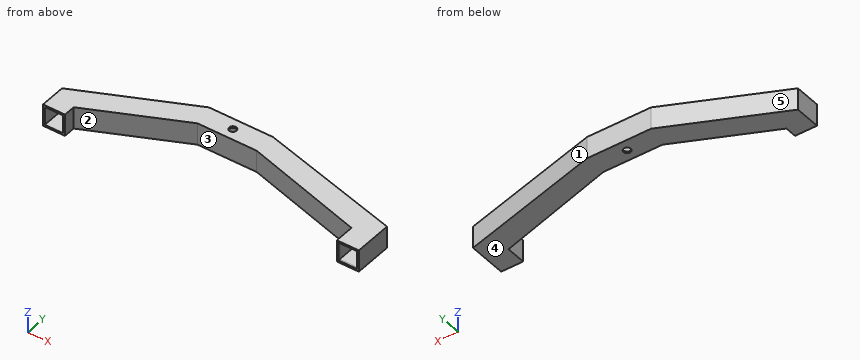
from build123d import *

# Parameters (mm, degrees)
BOSS_EXTRUDE1_DEPTH = 12
SHELL1_T            = -1
SKETCH2_W           = 10
SKETCH2_H           = 10
CUT_EXTRUDE1_DEPTH  = 12
SKETCH3_R           = 2
CUT_EXTRUDE2_DEPTH  = 12
CUT_EXTRUDE3_REACH  = 43.63
SKETCH5_W           = 0.21800788
SKETCH5_H           = 12


with BuildPart() as part:
    # Sketch1 → Boss-Extrude1 (new body)
    with BuildSketch(Plane.XY):
        Polygon((82.939086493, -35.63), (82.939086493, -24.776717085), (17.5, -6), (-14.870410096, -6), (-65.342905627, -29.23610302), (-65.342905627, -35.63), (-77.342905627, -35.63), (-77.342905627, -21.549973615), (-17.5, 6), (17.5, 6), (95.157094373, -14.812940234), (95.157094373, -35.63), align=None)
    extrude(amount=BOSS_EXTRUDE1_DEPTH)

    # Shell1
    shell1_openings = [part.faces().sort_by_distance(p)[0] for p in [
        (-71.342905627, -35.63, 6),
    ]]
    offset(amount=SHELL1_T, openings=shell1_openings, kind=Kind.INTERSECTION)

    # Sketch2 → Cut-Extrude1 (cut)
    with BuildSketch(Plane.XZ.offset(35.63)):
        with Locations((89.157094373, 6.101364163)):
            Rectangle(SKETCH2_W, SKETCH2_H)
    extrude(amount=-CUT_EXTRUDE1_DEPTH, mode=Mode.SUBTRACT)

    # Sketch3 → Cut-Extrude2 (cut)
    with BuildSketch(Plane.XY.offset(12)):
        Circle(SKETCH3_R)
    extrude(amount=-CUT_EXTRUDE2_DEPTH, mode=Mode.SUBTRACT)

    # Cut-Extrude3: up to this face of the body (flat: up to its plane)
    cut_extrude3_end = Plane(part.part.faces().sort_by_distance((50.219543247, -15.388358542, 6))[0])
    # Sketch5 → Cut-Extrude3 (cut, up to the picked face)
    with BuildSketch(Plane.XZ.offset(35.63), mode=Mode.PRIVATE) as cut_extrude3_sk1:
        with Locations((83.048090433, 6)):
            Rectangle(SKETCH5_W, SKETCH5_H)
    cut_extrude3_tool1 = split(extrude(cut_extrude3_sk1.sketch, amount=-CUT_EXTRUDE3_REACH, mode=Mode.PRIVATE), bisect_by=cut_extrude3_end, keep=Keep.BOTH, mode=Mode.PRIVATE)
    add(cut_extrude3_tool1.solids().sort_by_distance((83.04809, -35.63, 6))[0], mode=Mode.SUBTRACT)


solid = part.part
Source: CAD feature listing. Evaluate the final solid. Frame: model axes, mm. Face numbers are marked on the shaded views. A direction names the side the tool comes from. Give positions to 0.01 mm unless a question says otherwise; leave off trailing zeros. Write each loop counter-clockwise with the first axis right and the second up, starting at its lowest first coordinate (ties: lowest second). Pieces come first, ordered by that corner, then holes. Notation, with made-up numbers: (55.5, 61.5) -> (88.5, 61.5) arc R20 cw to (88.5, 71.5) -> close; hole circle Ø2 at (25.25, 16.25). An arc over 180 degrees is marked (long way). Return JSON: item names as keys, results as strings. Group by question number.
1. Section C-C, the plane z = 7. Output: boundary loops of the cut face in (x, y), then the cut area to 3 significant figures.
2. Section D-D, the plane y = -10. Output: boundary loops of the cut face in (x, z), then the cut area to 3 significant figures.
3. Material intervals for line 1 (Y direction, x = 0, z = 11.4); line 2 (Z direction, x = 54.5, y = -8.5); line 3 (X direction, y = -25, z = 2.75), sorted ascending. Write a range as from..to.
4. Access query for the marked faces 1 and 2. Directions: +Z, -Z, +X, -X, +Y, -Y. A direction counts if a zero-diameter tool reaches every point of the face in a straight line with its end or side. Return the directions, or none.
5. Pin query (flat end, axial travel): pin 1 Ø6 at (x, z) = (11, 7) entering from -Y; pin 2 Ø4 at (y, z) = (-9.5, 1.5) entering from -X; pin 3 Ø12 at (x, y) = (-1, -15) entering from +Z. Return the tip coordinate at first contact, or that it passes through.
6. Section A-A, the plane x = 0. Output: boundary loops of the cut face in (y, z).
7. Mould query, pull axis X, two halves, no side actions, for the marked faces 3, 4 and 5. Classes: +X half, -X half, draft (parallel to the pull), parting line (faces both ways), or undercut.
8. Section B-B, the plane y = 0. Output: boundary loops of the cut face in (x, z).
Determined:
{
 "1": {"outline": "(-77.34, -35.63) -> (-76.34, -35.63) -> (-76.34, -22.19) -> (-17.28, 5) -> (17.37, 5) -> (94.16, -15.58) -> (94.16, -35.63) -> (95.16, -35.63) -> (95.16, -14.81) -> (17.5, 6) -> (-17.5, 6) -> (-77.34, -21.55) -> close; (-66.34, -35.63) -> (-65.34, -35.63) -> (-65.34, -29.24) -> (-14.87, -6) -> (17.5, -6) -> (83.16, -24.84) -> (83.16, -35.63) -> (84.16, -35.63) -> (84.16, -34.63) -> (83.94, -34.63) -> (83.94, -24.02) -> (17.64, -5) -> (-15.09, -5) -> (-66.34, -28.6) -> close", "area": "387 mm2"},
 "2": {"outline": "(-52.25, 0) -> (-23.56, 0) -> (-23.56, 12) -> (-52.25, 12) -> close; (31.44, 0) -> (77.2, 0) -> (77.2, 12) -> (31.44, 12) -> close; hole (-49.86, 1) -> (-25.95, 1) -> (-25.95, 11) -> (-49.86, 11) -> close; hole (35.07, 1) -> (73.34, 1) -> (73.34, 11) -> (35.07, 11) -> close", "area": "272 mm2"},
 "3": {"line 1": "y = -6..-2, 2..6", "line 2": "z = 0..1, 11..12", "line 3": "x = -77.34..-76.34, -58.53..-56.14, 83.16..83.94, 94.16..95.16"},
 "4": {"face 1": "+Z, -Z, +X, +Y", "face 2": "+Z, -Z, -Y"},
 "5": {"pin 1": "stops at y = -6", "pin 2": "stops at x = -55.51", "pin 3": "passes through"},
 "6": {"outline": "(-6, 0) -> (-2, 0) -> (-2, 1) -> (-5, 1) -> (-5, 11) -> (-2, 11) -> (-2, 12) -> (-6, 12) -> close; (2, 0) -> (6, 0) -> (6, 12) -> (2, 12) -> (2, 11) -> (5, 11) -> (5, 1) -> (2, 1) -> close"},
 "7": {"face 3": "undercut", "face 4": "draft", "face 5": "-X half"},
 "8": {"outline": "(-30.53, 0) -> (-2, 0) -> (-2, 1) -> (-28.14, 1) -> (-28.14, 11) -> (-2, 11) -> (-2, 12) -> (-30.53, 12) -> close; (2, 0) -> (39.89, 0) -> (39.89, 12) -> (2, 12) -> (2, 11) -> (36.02, 11) -> (36.02, 1) -> (2, 1) -> close"}
}
